The model under review builds one solid part; all positions refer to its coordinate system, in mm. A direction names the side the tool comes from. Give positions to 0.01 mm unless a question says otherwise; leave off trailing zeros. Write each loop counter-clockwise with the first axis right and the second up, starting at its lowest first coordinate (ties: lowest second). Pieces come first, ordered by that corner, then holes. Notation, with made-up numbers: (-38.75, 6.25) - (-4.75, 6.25) arc R4 ccw to (-4.75, 10.25) - close; hole circle Ø4 at (81, -12). An arc over 180 degrees is marked (long way). Write item = value, one per line.
```python
from build123d import *
from OCP.BRepFilletAPI import BRepFilletAPI_MakeChamfer

# Parameters (mm, degrees)
SKETCH1_R           = 3.5
BOSS_EXTRUDE1_DEPTH = 18
SKETCH2_W           = 9
SKETCH2_H           = 2
BOSS_EXTRUDE3_DEPTH = 10
CUT_EXTRUDE3_START  = -8
SKETCH3_W           = 10
SKETCH3_H           = 2.5
CUT_EXTRUDE3_DEPTH  = 4
CHAMFER1_SIZE       = 1
CHAMFER1_SIZE2      = 0.577350269


with BuildPart() as part:
    # Sketch1 → Boss-Extrude1 (new body)
    with BuildSketch(Plane(origin=(0, 0, 0), x_dir=(1, 0, 0), z_dir=(0, 1, 0))):
        with Locations(Location((0, 0, 0), (0, 0, 270))):
            Circle(SKETCH1_R)
    extrude(amount=BOSS_EXTRUDE1_DEPTH)

    # Sketch2 → Boss-Extrude3 (add)
    with BuildSketch(Plane(origin=(0, 18, 0), x_dir=(1, 0, 0), z_dir=(0, 1, 0))):
        Rectangle(SKETCH2_W, SKETCH2_H)
    extrude(amount=-BOSS_EXTRUDE3_DEPTH)

    # Sketch3 → Cut-Extrude3 (cut)
    with BuildSketch(Plane.XZ.offset(CUT_EXTRUDE3_START)):
        with Locations((0, -2.25)):
            Rectangle(SKETCH3_W, SKETCH3_H)
    extrude(amount=-CUT_EXTRUDE3_DEPTH, mode=Mode.SUBTRACT)

    # Chamfer1: one chamfer whose edges measure the first distance from different faces: ONE call of the kernel's chamfer builder (chamfer() names one face for all edges)
    chamfer1_edges_1 = [part.edges().sort_by_distance(p)[0] for p in [
        (3.927050983, 18, -1),
        (-3.927050983, 18, -1),
    ]]
    chamfer1_side_1 = [part.faces().sort_by_distance(p)[0] for p in [
        (0, 11.381966011, -1),
    ]]
    chamfer1_edges_2 = [part.edges().sort_by_distance(p)[0] for p in [
        (3.927050983, 18, 1),
    ]]
    chamfer1_side_2 = [part.faces().sort_by_distance(p)[0] for p in [
        (3.927050983, 13, 1),
    ]]
    chamfer1_edges_3 = [part.edges().sort_by_distance(p)[0] for p in [
        (4.5, 18, 0),
    ]]
    chamfer1_side_3 = [part.faces().sort_by_distance(p)[0] for p in [
        (4.5, 13, 0),
    ]]
    chamfer1_edges_4 = [part.edges().sort_by_distance(p)[0] for p in [
        (-3.927050983, 18, 1),
    ]]
    chamfer1_side_4 = [part.faces().sort_by_distance(p)[0] for p in [
        (-3.927050983, 13, 1),
    ]]
    chamfer1_edges_5 = [part.edges().sort_by_distance(p)[0] for p in [
        (-4.5, 18, 0),
    ]]
    chamfer1_side_5 = [part.faces().sort_by_distance(p)[0] for p in [
        (-4.5, 13, 0),
    ]]
    chamfer1_edges_6 = [part.edges().sort_by_distance(p)[0] for p in [
        (0, 18, -3.5),
    ]]
    chamfer1_side_6 = [part.faces().sort_by_distance(p)[0] for p in [
        (0, 15, -3.5),
    ]]
    chamfer1_edges_7 = [part.edges().sort_by_distance(p)[0] for p in [
        (2.091650066, 18, 2.80624304),
    ]]
    chamfer1_side_7 = [part.faces().sort_by_distance(p)[0] for p in [
        (0, 9, -3.5),
    ]]
    chamfer1 = BRepFilletAPI_MakeChamfer(part.part.solid().wrapped)
    for e in chamfer1_edges_1:
        chamfer1.Add(CHAMFER1_SIZE, CHAMFER1_SIZE2, e.wrapped, chamfer1_side_1[0].wrapped)  # the first distance lies on this face
    for e in chamfer1_edges_2:
        chamfer1.Add(CHAMFER1_SIZE, CHAMFER1_SIZE2, e.wrapped, chamfer1_side_2[0].wrapped)  # the first distance lies on this face
    for e in chamfer1_edges_3:
        chamfer1.Add(CHAMFER1_SIZE, CHAMFER1_SIZE2, e.wrapped, chamfer1_side_3[0].wrapped)  # the first distance lies on this face
    for e in chamfer1_edges_4:
        chamfer1.Add(CHAMFER1_SIZE, CHAMFER1_SIZE2, e.wrapped, chamfer1_side_4[0].wrapped)  # the first distance lies on this face
    for e in chamfer1_edges_5:
        chamfer1.Add(CHAMFER1_SIZE, CHAMFER1_SIZE2, e.wrapped, chamfer1_side_5[0].wrapped)  # the first distance lies on this face
    for e in chamfer1_edges_6:
        chamfer1.Add(CHAMFER1_SIZE, CHAMFER1_SIZE2, e.wrapped, chamfer1_side_6[0].wrapped)  # the first distance lies on this face
    for e in chamfer1_edges_7:
        chamfer1.Add(CHAMFER1_SIZE, CHAMFER1_SIZE2, e.wrapped, chamfer1_side_7[0].wrapped)  # the first distance lies on this face
    add(Compound.cast(chamfer1.Shape()), mode=Mode.REPLACE)


solid = part.part
```
1. Take a section at C-C on z = 0. Give the boundary of the cut face in (x, y), and give its area (3 significant figures).
Findings below:
outline = (-4.5, 8) - (-3.5, 8) - (-3.5, 0) - (3.5, 0) - (3.5, 8) - (4.5, 8) - (4.5, 17) - (3.92, 18) - (-3.92, 18) - (-4.5, 17) - close
area = 145 mm²
2. Machinability: for faces 1 (the flat face through (3.685, 17.507, 0.707)), 2 (the flat face through (3.685, 17.507, -0.707)), 3 (the flat face through (-3.707, 17.507, -0.707)), 4 (the flat face through (0, 8, -2)), which of the approach directions +Z, -Z, +X, -X, +Y, -Y give a long, thin tool a straight path to every point of the face, cutting with its end or side? Answer none if there is none.
Findings below:
face_1 = +Z, +X, +Y
face_2 = -Z, +X, +Y
face_3 = -Z, -X, +Y
face_4 = -Z, +X, -X
3. Take a section at B-B on y = 16.25. Give the boundary of the cut face in (x, z).
Findings below:
outline = (-4.5, -1) - (-3.35, -1) arc R3.5 ccw to (3.35, -1) - (4.5, -1) - (4.5, 1) - (3.35, 1) arc R3.5 ccw to (-3.35, 1) - (-4.5, 1) - close
4. For line 1 (Y direction, x = -2, z = -1.5); line 2 (X direction, y = 5.75, z = 0); line 3 (Z direction, x = 1, y = 15.75), list the stretches that pass through material, from the lowest coordinate up. Write a range as from..to.
Findings below:
line_1 = 0..8, 12..18
line_2 = -3.5..3.5
line_3 = -3.35..3.35
5. Insertion check: P1, Ø3, axis at x = 1.5, y = 14.5, coming from the +Z side; P2, Ø3, axis at y = 6.5, z = -1.5, coming from the -X side; P3, Ø0.6, axis at x = -3.5, y = 11, coming from the +Z side; P4, Ø2, axis at x = 3.5, y = 5, coming from the +Z side. Each pin has a flat end and moves straight along its axis. Give the tip position at first contact, or say it passes through.
Findings below:
P1 = 3.5
P2 = -3.5
P3 = 1.42
P4 = 2.45
6. Draft analysis for pull direction Y (two halves, no side actions). For faces 5 (the conical face through (0.06, 17.84, -3.014)), 6 (the flat face through (-4, 13, 1)), 7 (the flat face through (0, 12, -2)), state which applies: +Y half, -Y half, draft (parallel to the pull), parting line (faces both ways), or undercut.
Findings below:
face_5 = +Y half
face_6 = draft
face_7 = undercut
7. Take a section at D-D on x = 3.75. Give the boundary of the cut face in (y, z), and give its area (3 significant figures).
Findings below:
outline = (8, -1) - (17, -1) - (18, -0.42) - (18, 0.42) - (17, 1) - (8, 1) - close
area = 19.4 mm²
8. Take a section at A-A on x = 0. Give the boundary of the cut face in (y, z).
Findings below:
outline = (0, -3.5) - (8, -3.5) - (8, -1) - (12, -1) - (12, -3.5) - (17, -3.5) - (18, -2.92) - (18, 2.92) - (17, 3.5) - (0, 3.5) - close
